CAD build for the part. Positions are in the model's coordinates, mm. Coordinates: 2 decimals unless noted, no trailing zeros. Loops run counter-clockwise (first coordinate to the right, second up) from the corner with the lowest first, then second, coordinate; pieces in that order, holes last. Notation, with made-up numbers: (-37, 48) -> (19, 48) arc R35 ccw to (19, 87) -> close; hole circle Ø4 at (56, -3.75). An arc over 180 degrees is marked (long way). Answer as a JSON object with one key per item and string values. Group by question number.
from build123d import *

# Parameters (mm, degrees)
F2_R     = 4.7625
F3_DEPTH = 19.05


with BuildPart() as f3:
    # F2 (on Right) → F3 (new body)
    with BuildSketch(Plane.YZ):
        with BuildLine():
            ThreePointArc((-749.54648, 275.423549), (-768.813366, 256.592933), (-749.98275, 237.326046))
            Line((-749.98275, 237.326046), (-602.102315, 235.632607))
            ThreePointArc((-602.102315, 235.632607), (-584.771859, 242.194496), (-576.511176, 258.78257))
            Line((-576.511176, 258.78257), (-541.569312, 651.973339))
            ThreePointArc((-541.569312, 651.973339), (-558.858252, 672.634838), (-579.519752, 655.345898))
            Line((-579.519752, 655.345898), (-607.177403, 344.122272))
            ThreePointArc((-607.177403, 344.122272), (-631.959454, 294.358051), (-683.950822, 274.672386))
            Line((-683.950822, 274.672386), (-749.54648, 275.423549))
        make_face()
        with Locations((-749.764615, 256.374798)):
            Circle(F2_R, mode=Mode.SUBTRACT)
        with Locations((-601.811469, 261.030942)):
            Circle(F2_R, mode=Mode.SUBTRACT)
        with Locations((-560.544532, 653.659618)):
            Circle(F2_R, mode=Mode.SUBTRACT)
    extrude(amount=F3_DEPTH)


solid = f3.part
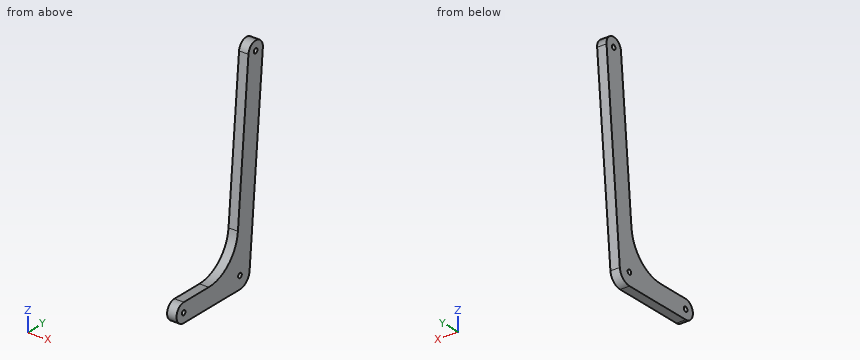
Item 1: Band-saw the part on B-B, the plane z = 305.5. List the corners of the cut face in (x, y), and give its area (3 significant figures).
Item 2: Band-saw the part on A-A, the plane x = 6. Count the separate pieces of the cut face and the enclosed holes in it, and give its area (3 significant figures).
Item 3: Flat gauge pins, fed straight in: P1, Ø4, axis at x = 17, z = 605.5, coming from the +Y side; P2, Ø1.5, axis at x = 10, y = -635.5, coming from the -Z side; P3, Ø3, axis at x = 8, y = -642, coming from the -Z side; P4, Ø7.5, axis at y = -560.54, z = 653.66, coming from the +X side. Where does each tip first touch, or does it go through?
Item 4: Band-saw the part on C-C, the plane y = -709.5. List the corners of the cut face in (x, z), and give its area (3 significant figures).
Item 5: Drill centre lines: L1, parallel to Z at x = 7.25, y = -743; L2, parallel to Y at x = 17.75, z = 654; L3, parallel to Y at x = 12.5, z = 319. Where is each one in solid material? Low to high.
Reply:
{
 "1": {"outline": "(0, -621.86) -> (19.05, -621.86) -> (19.05, -572.36) -> (0, -572.36) -> close", "area": "943 mm²"},
 "2": {"separate pieces": "1", "enclosed holes": "3", "area": "23,000 mm²"},
 "3": {"P1": "y = -545.52", "P2": "z = 236.01", "P3": "z = 236.07", "P4": "through"},
 "4": {"outline": "(0, 236.86) -> (19.05, 236.86) -> (19.05, 274.96) -> (0, 274.96) -> close", "area": "726 mm²"},
 "5": {"L1": "237.25 to 275.35", "L2": "-579.64 to -565.29, -555.79 to -541.5", "L3": "-613.86 to -571.16"}
}
